Verification items for this drawing (mm, ordinates from the low corner). Coordinates: 2 decimals unless noted, no trailing zeros. Order: outer loops, then holes, each group sorted by start corner. A loop starts at its lowest first (then second) coordinate and runs counter-clockwise, first axis right, second up. Notation, with made-up numbers: M -29,69.25 L 21,69.25 A20 cw 21,93.25 Z; hole C 39,14.5 d2. An arc over 180 degrees is marked long. Write item = value, one per line.
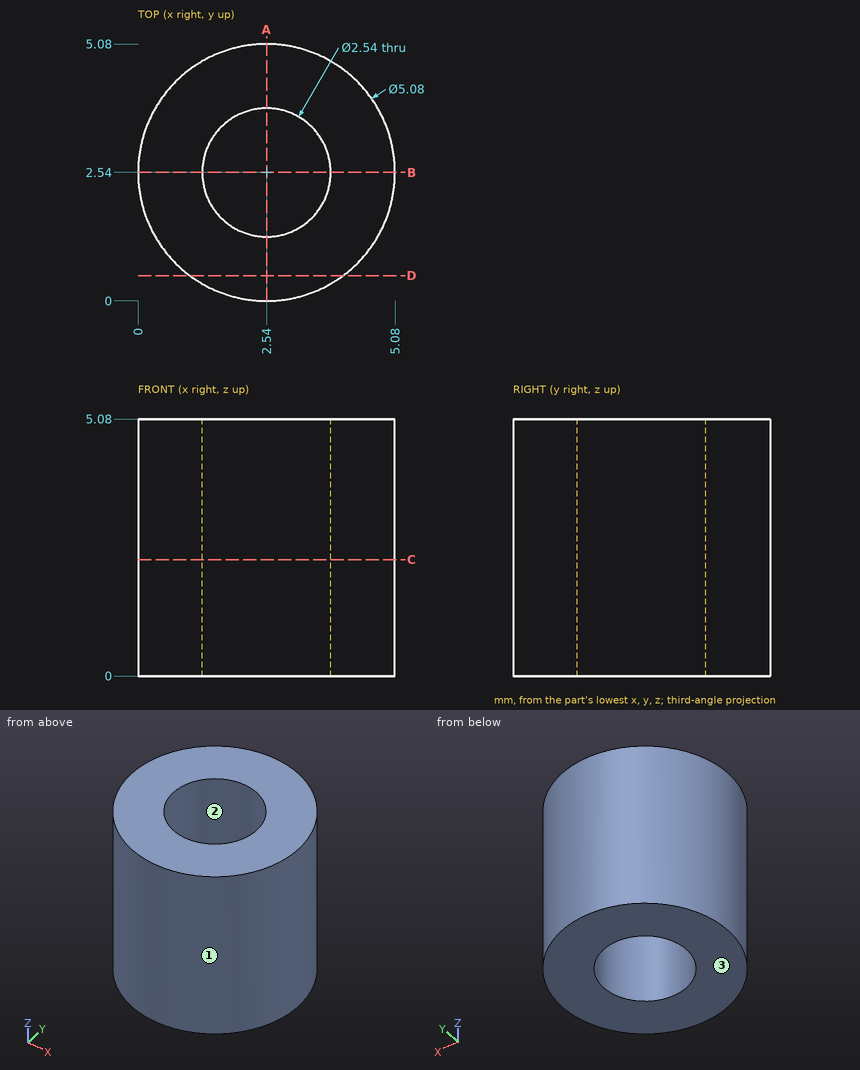
Item 1: Sectioned sample at C-C, the plane z = 2.3. Enter the section's corners in (x, y).
Report:
outline = C 2.54,2.54 d5.08; hole C 2.54,2.54 d2.54
Item 2: Sectioned sample at D-D, the plane y = 0.5. Enter the section's corners in (x, z), then the cut area to 3 significant figures.
Report:
outline = M 1.03,0 L 4.05,0 L 4.05,5.08 L 1.03,5.08 Z
area = 15.4 mm^2
Item 3: Scan lines: L1, parallel to Y at x = 2.55, z = 0.65; L2, parallel to Y at x = 3.2, z = 1.55; L3, parallel to Y at x = 4.8, z = 2.7. Record each from-to range of solid material in increasing order. Write a range as from..to.
Report:
L1 = 0..1.27, 3.81..5.08
L2 = 0.09..1.45, 3.63..4.99
L3 = 1.38..3.7
Item 4: Release check for a two-part mould opening along X. For the marked faces 1, 2 and 3 record: pulls with the +X half, pulls with the -X half, needs draft (parallel to the pull), parting line crosses it, or undercut.
Report:
face_1 = parting line crosses it
face_2 = undercut
face_3 = needs draft
Item 5: Sectioned sample at A-A, the plane x = 2.54. Enter the section's corners in (y, z), then the cut area to 3 significant figures.
Report:
outline = M 0,0 L 1.27,0 L 1.27,5.08 L 0,5.08 Z; M 3.81,0 L 5.08,0 L 5.08,5.08 L 3.81,5.08 Z
area = 12.9 mm^2
Item 6: Gauge pin test, flat ends, axial feed: pin 1 (3 mm diameter, centred on x = 2.54, y = 2.54, fed in from -Z); pin 2 (3 mm diameter, centred on y = 4.5, z = 1, fed in from +X). Record the tip position at first contact, or that the pin passes through.
Report:
pin_1 = 0
pin_2 = 5.04
